CAD build for the part. Positions are in the model's coordinates, mm. A direction names the side the tool comes from. Coordinates: 2 decimals unless noted, no trailing zeros. Write each loop counter-clockwise with the first axis right and the second up, starting at its lowest first coordinate (ties: lowest second). Pieces come first, ordered by that corner, then holes. Notation, with made-up numbers: (49.25, -8.75) - (87.25, -8.75) arc R23 cw to (87.25, 26.25) - close; hole circle Ø7 at (-13, -26). An arc over 180 degrees is marked (long way). One line per question, with ' | ' between items. Start each with the question number.
1. Band-saw the part on A-A, the plane y = 64.5. Write the cut outline in (x, z).
2. Which spindle directions (+Z, -Z, +X, -X, +Y, -Y) get a long thin tool onto all of the face, cutting with end or side? Do faces 1 (the flat face through (318, -22, 110)), 2 (the flat face through (351, 183, 10)). Say none if no direction does.
3. Flat gauge pins, fed straight in: P1, Ø3, axis at x = 357.07, z = 60, coming from the +Y side; P2, Ø1, axis at x = 249.5, y = 25, coming from the +Z side. Where does each tip first touch, or does it go through?
4. Two-plate mould, pull along Y, no slides. Class faces 3 (the flat face through (350, 430.1, 54)), 4 (the flat face through (-92.926, 177, 61)), 5 (the flat face through (857.074, 177, 54)): +Y half, -Y half, draft (parallel to the pull), parting line (faces both ways), or undercut.
5. Band-saw the part on C-C, the plane x = -45.5. Write the cut outline in (y, z).
6. Band-saw the part on B-B, the plane z = 27. Write the cut outline in (x, y).
7. Probe line 1 (X direction, y = 349, z = 56.5); line 2 (Y direction, x = 123.5, z = 34); line 3 (Z direction, x = 664.5, y = 104.5). List the from-to ranges inside material, lowest first.
from build123d import *

# Parameters (mm, degrees)
F0_W      = 1000
F0_H      = 500
F1_DEPTH  = 110
F2_W      = 900
F2_H      = 400
F3_DEPTH  = 100
F5_DEPTH  = 50
F6_R      = 2.5
F7_DEPTH  = 50
F8_R      = 2.5
F9_DEPTH  = 25
F10_DEPTH = 25
F11_R     = 2.5
F12_DEPTH = 25


with BuildPart() as f1:
    # F0 (on Top) → F1 (new body)
    with BuildSketch(Plane.XY):
        with Locations((357.0744521916, 180.0998109607)):
            Rectangle(F0_W, F0_H)
    extrude(amount=F1_DEPTH)

    # F2 (on face) → F3 (cut)
    with BuildSketch(Plane.XY.offset(110)):
        with Locations((357.0744521916, 180.0998109607)):
            Rectangle(F2_W, F2_H)
    extrude(amount=-F3_DEPTH, mode=Mode.SUBTRACT)

    # F4 (on face) → F5 (cut)
    with BuildSketch(Plane.XZ.offset(-380.0998109607)):
        with BuildLine():
            ThreePointArc((359.5744521916, 60), (358.8422191446, 61.767766953), (357.0744521916, 62.5))
            Line((357.0744521916, 62.5), (357.0744521916, 57.5))
            ThreePointArc((357.0744521916, 57.5), (358.8422191446, 58.232233047), (359.5744521916, 60))
        make_face()
        with BuildLine():
            Line((357.0744521916, 57.5), (357.0744521916, 62.5))
            ThreePointArc((357.0744521916, 62.5), (354.5744521916, 60), (357.0744521916, 57.5))
        make_face()
    extrude(amount=-F5_DEPTH, mode=Mode.SUBTRACT)

    # F6 (on face) → F7 (cut)
    with BuildSketch(Plane(origin=(0, -19.9001890393, 0), x_dir=(-1, 0, 0), z_dir=(0, 1, 0))):
        with Locations((-357.0744521916, 60)):
            Circle(F6_R)
    extrude(amount=-F7_DEPTH, mode=Mode.SUBTRACT)

    # F8 (on face) → F9 (cut)
    with BuildSketch(Plane.XZ.offset(-380.0998109607)):
        with Locations((132.0744521916, 60)):
            Circle(F8_R)
    extrude(amount=-F9_DEPTH, mode=Mode.SUBTRACT)

    # F8 (on face) → F10 (cut)
    with BuildSketch(Plane.XZ.offset(-380.0998109607)):
        with Locations((132.0744521916, 60)):
            Circle(F8_R)
        with Locations((582.0744521916, 60)):
            Circle(F8_R)
    extrude(amount=-F10_DEPTH, mode=Mode.SUBTRACT)

    # F11 (on face) → F12 (cut)
    with BuildSketch(Plane(origin=(0, -19.9001890393, 0), x_dir=(-1, 0, 0), z_dir=(0, 1, 0))):
        with Locations((-132.0744521916, 60)):
            Circle(F11_R)
        with Locations((-582.0744521916, 60)):
            Circle(F11_R)
    extrude(amount=-F12_DEPTH, mode=Mode.SUBTRACT)


solid = f1.part
Filled in:
1) outline: (-142.93, 0) - (857.07, 0) - (857.07, 110) - (807.07, 110) - (807.07, 10) - (-92.93, 10) - (-92.93, 110) - (-142.93, 110) - close
2) face 1: +Z, +X, -X, +Y, -Y | face 2: +Z
3) P1: passes through | P2: stops at z = 10
4) face 3: +Y half | face 4: undercut | face 5: draft
5) outline: (-69.9, 0) - (430.1, 0) - (430.1, 110) - (380.1, 110) - (380.1, 10) - (-19.9, 10) - (-19.9, 110) - (-69.9, 110) - close
6) outline: (-142.93, -69.9) - (857.07, -69.9) - (857.07, 430.1) - (-142.93, 430.1) - close; hole (-92.93, -19.9) - (807.07, -19.9) - (807.07, 380.1) - (-92.93, 380.1) - close
7) line 1: x = -142.93 to -92.93, 807.07 to 857.07 | line 2: y = -69.9 to -19.9, 380.1 to 430.1 | line 3: z = 0 to 10
